Check sheet for the modelled part. Datum: model origin and axes. Units: mm. A direction names the side the tool comes from. Round coordinates to 2 decimals unless told otherwise and drop trailing zeros. Loops run counter-clockwise (first coordinate to the right, second up) from the corner with the lowest first, then second, coordinate; pieces in that order, holes last. Notation, with made-up numbers: (52, -2.5) - (93, -2.5) arc R24 cw to (93, 13.5) - close; hole circle Ø6 at (-35, 59). An arc over 180 degrees is marked (long way). Put each result on its own line as item: value.
```python
from build123d import *

# Parameters (mm, degrees)
F0_W     = 63.5
F0_H     = 50.8
F1_DEPTH = 63.5
F2_W     = 25.3320866376
F2_H     = 25.1011773944
F2_W_2   = 12.7
F2_H_2   = 63.5
F3_DEPTH = 25.4
F4_W     = 12.7
F4_H     = 15.8308558166
F5_DEPTH = 25.4


with BuildPart() as f1:
    # F0 (on Front) → F1 (new body)
    with BuildSketch(Plane.XZ):
        with Locations((10.4112830013, -5.1873601034)):
            Rectangle(F0_W, F0_H)
    extrude(amount=F1_DEPTH)

    # F2 (on face) → F3 (cut)
    with BuildSketch(Plane.XY.offset(20.2126398966)):
        with Locations((29.4952396825, -39.2205901444)):
            Rectangle(F2_W, F2_H)
        with Locations((-9.9087147206, -31.75)):
            Rectangle(F2_W_2, F2_H_2)
    extrude(amount=-F3_DEPTH, mode=Mode.SUBTRACT)

    # F4 (on face) → F5 (join)
    with BuildSketch(Plane.XY.offset(-5.1873601034)):
        with Locations((-9.9087147206, -7.9154279083)):
            Rectangle(F4_W, F4_H)
    extrude(amount=F5_DEPTH)


solid = f1.part
```
Item 1: Go/stop test with flat-tipped pins: pin 1 (7.5 mm diameter, centred on y = -34.5, z = 12, fed in from +X); pin 2 (12 mm diameter, centred on x = 23, y = -41.5, fed in from +Z). Record where each tip stops, or that it passes through.
Filled sheet:
pin 1: x = 16.83
pin 2: z = -5.19
Item 2: Section check B-B on z = 5. Enter the section's corners in (x, y), then the cut area to 3 significant figures.
Filled sheet:
outline: (-21.34, -63.5) - (-16.26, -63.5) - (-16.26, -15.83) - (-3.56, -15.83) - (-3.56, -63.5) - (42.16, -63.5) - (42.16, -51.77) - (16.83, -51.77) - (16.83, -26.67) - (42.16, -26.67) - (42.16, 0) - (-21.34, 0) - close
area: 2,790 mm²
Item 3: Section check C-C on x = 30. Enter the section's corners in (y, z).
Filled sheet:
outline: (-63.5, -30.59) - (0, -30.59) - (0, 20.21) - (-26.67, 20.21) - (-26.67, -5.19) - (-51.77, -5.19) - (-51.77, 20.21) - (-63.5, 20.21) - close
Item 4: Release check for a two-part mould opening along X. For faces 4 (the flat face through (10, -31, 20.213)), 5 (the flat face through (-10, -15.831, 7)), 6 (the flat face through (16.829, -39, 8)) record: +X half, -X half, draft (parallel to the pull), parting line (faces both ways), or undercut.
Filled sheet:
face 4: draft
face 5: undercut
face 6: +X half
Item 5: Thickness scan on line 1 (X direction, y = -16.5, z = -3); line 2 (X direction, y = -33, z = 0.5); line 3 (Y direction, x = 24.5, z = -3). Record the ranges inside material, lowest first. Write a range as from..to.
Filled sheet:
line 1: -21.34..-16.26, -3.56..42.16
line 2: -21.34..-16.26, -3.56..16.83
line 3: -63.5..-51.77, -26.67..0
Item 6: Tool access check on faces 1 (the flat face through (-10, -39, -5.187)), 2 (the flat face through (29, -51.771, 8)), 3 (the flat face through (42.161, -31, -6)). Record the directions out of +Z, -Z, +X, -X, +Y, -Y that give a thin tool (end or side, any length) a straight path to the whole face; none if there is none.
Filled sheet:
face 1: +Z, -Y
face 2: +Z, +X
face 3: +Z, -Z, +X, +Y, -Y
Item 7: Section check D-D on y = -50. Enter the section's corners in (x, z), then the cut area to 3 significant figures.
Filled sheet:
outline: (-21.34, -30.59) - (42.16, -30.59) - (42.16, -5.19) - (16.83, -5.19) - (16.83, 20.21) - (-3.56, 20.21) - (-3.56, -5.19) - (-16.26, -5.19) - (-16.26, 20.21) - (-21.34, 20.21) - close
area: 2,260 mm²
Item 8: Section check A-A on y = -19.5. Enter the section's corners in (x, z).
Filled sheet:
outline: (-21.34, -30.59) - (42.16, -30.59) - (42.16, 20.21) - (-3.56, 20.21) - (-3.56, -5.19) - (-16.26, -5.19) - (-16.26, 20.21) - (-21.34, 20.21) - close
